Work out the finished part from the listing and answer in its coordinate system (mm). A direction names the side the tool comes from. Round coordinates to 2 decimals unless told otherwise and drop trailing zeros. Loops run counter-clockwise (first coordinate to the right, second up) from the corner with the lowest first, then second, coordinate; pieces in that order, holes last. Notation, with made-up numbers: (25, -37) -> (72, -37) arc R20 ccw to (72, -14) -> close; hole circle Ø7 at (-16.75, 11). An arc over 180 degrees is marked (long way). Use one line per item in the form item = value.
```python
from build123d import *

# Parameters (mm, degrees)
ESQUISSE1_W        = 49.7
ESQUISSE1_H        = 55.3
ESQUISSE1_R        = 2
BOSS_EXTRU_1_DEPTH = 1.5
CONG_1_R           = 1
ESQUISSE2_W        = 24
ESQUISSE2_H        = 10.127456192
BOSS_EXTRU_2_DEPTH = 25
ESQUISSE3_W        = 7.5
ESQUISSE3_H        = 10.5
BOSS_EXTRU_3_DEPTH = 10
ESQUISSE4_W        = 15
ESQUISSE4_H        = 8
BOSS_EXTRU_4_DEPTH = 10
ESQUISSE5_W        = 8
ESQUISSE5_H        = 8
BOSS_EXTRU_5_DEPTH = 8


with BuildPart() as part:
    # Esquisse1 → Boss.-Extru.1 (new body)
    with BuildSketch(Plane.XY):
        with Locations((24.85, 27.65)):
            Rectangle(ESQUISSE1_W, ESQUISSE1_H)
        with Locations((3.6, 51.7)):
            Circle(ESQUISSE1_R, mode=Mode.SUBTRACT)
        with Locations((46.1, 51.7)):
            Circle(ESQUISSE1_R, mode=Mode.SUBTRACT)
        with Locations((46.1, 3.6)):
            Circle(ESQUISSE1_R, mode=Mode.SUBTRACT)
        with Locations((3.6, 3.6)):
            Circle(ESQUISSE1_R, mode=Mode.SUBTRACT)
    extrude(amount=BOSS_EXTRU_1_DEPTH)

    # Congé1
    cong_1_edges = [part.edges().sort_by_distance(p)[0] for p in [
        (0, 55.3, 0.75),
        (49.7, 55.3, 0.75),
        (49.7, 0, 0.75),
        (0, 0, 0.75),
    ]]
    fillet(cong_1_edges, radius=CONG_1_R)

    # Esquisse2 → Boss.-Extru.2 (add)
    with BuildSketch(Plane.XY.offset(1.5)):
        with Locations((24.85, 50.236271904)):
            Rectangle(ESQUISSE2_W, ESQUISSE2_H)
    extrude(amount=BOSS_EXTRU_2_DEPTH)

    # Esquisse3 → Boss.-Extru.3 (add)
    with BuildSketch(Plane.XY.offset(1.5)):
        with Locations((3.75, 17.25)):
            Rectangle(ESQUISSE3_W, ESQUISSE3_H)
        with Locations((45.95, 17.25)):
            Rectangle(ESQUISSE3_W, ESQUISSE3_H)
    extrude(amount=BOSS_EXTRU_3_DEPTH)

    # Esquisse4 → Boss.-Extru.4 (add)
    with BuildSketch(Plane.XY.offset(1.5)):
        with Locations((24.85, 5)):
            Rectangle(ESQUISSE4_W, ESQUISSE4_H)
    extrude(amount=BOSS_EXTRU_4_DEPTH)

    # Esquisse5 → Boss.-Extru.5 (add)
    with BuildSketch(Plane.XY.offset(1.5)):
        with Locations((36.35, 5)):
            Rectangle(ESQUISSE5_W, ESQUISSE5_H)
    extrude(amount=BOSS_EXTRU_5_DEPTH)


solid = part.part
```
(1) Find section B-B, the plane y = 51.7. Write down the section's boundary in (x, z), then the cut area to 3 significant figures.
Completed:
outline = (0, 0) -> (1.6, 0) -> (1.6, 1.5) -> (0, 1.5) -> close; (5.6, 0) -> (44.1, 0) -> (44.1, 1.5) -> (36.85, 1.5) -> (36.85, 26.5) -> (12.85, 26.5) -> (12.85, 1.5) -> (5.6, 1.5) -> close; (48.1, 0) -> (49.7, 0) -> (49.7, 1.5) -> (48.1, 1.5) -> close
area = 663 mm2
(2) For faces 5 (the flat face through (4, 22.5, 6)), 6 (the flat face through (29, 9, 6)), 7 (the flat face through (12.85, 50, 14)), determine the directions among +Z, -Z, +X, -X, +Y, -Y from which every point of the face is accessible in a straight line to the end or side of a thin tool.
Completed:
face_5 = +Z, +X, -X, +Y
face_6 = +Z, +X, -X
face_7 = +Z, -X, +Y, -Y
(3) Find section D-D, the plane x = 28. Write down the section's boundary in (y, z), then the cut area to 3 significant figures.
Completed:
outline = (0, 0) -> (55.3, 0) -> (55.3, 26.5) -> (45.17, 26.5) -> (45.17, 1.5) -> (9, 1.5) -> (9, 11.5) -> (1, 11.5) -> (1, 1.5) -> (0, 1.5) -> close
area = 416 mm2
(4) Consider L1, parallel to Y at x = 46.1, z = 0.9; L2, parallel to X at y = 18, z = 9.5; L3, parallel to Y at x = 32, z = 19.25. Determine where each line is inside the solid, lowest interval first.
Completed:
L1 = 0 to 1.6, 5.6 to 49.7, 53.7 to 55.3
L2 = 0 to 7.5, 42.2 to 49.7
L3 = 45.17 to 55.3
(5) Find section C-C, the plane z = 10.5. Write down the section's boundary in (x, y).
Completed:
outline = (0, 12) -> (7.5, 12) -> (7.5, 22.5) -> (0, 22.5) -> close; (12.85, 45.17) -> (36.85, 45.17) -> (36.85, 55.3) -> (12.85, 55.3) -> close; (17.35, 1) -> (32.35, 1) -> (32.35, 9) -> (17.35, 9) -> close; (42.2, 12) -> (49.7, 12) -> (49.7, 22.5) -> (42.2, 22.5) -> close
(6) For a pull along Y with two mould halves and no side action, classify faces 1 (the flat face through (46, 12, 6)), 2 (the flat face through (46, 22.5, 6)), 3 (the flat face through (25, 28, 1.5)), 4 (the flat face through (42.2, 17, 6)) as +Y half, -Y half, draft (parallel to the pull), parting line (faces both ways), or undercut.
Completed:
face_1 = -Y half
face_2 = +Y half
face_3 = undercut
face_4 = draft
(7) Find section A-A, the plane x = 46.1. Write down the section's boundary in (y, z), then the cut area to 3 significant figures.
Completed:
outline = (0, 0) -> (1.6, 0) -> (1.6, 1.5) -> (0, 1.5) -> close; (5.6, 0) -> (49.7, 0) -> (49.7, 1.5) -> (22.5, 1.5) -> (22.5, 11.5) -> (12, 11.5) -> (12, 1.5) -> (5.6, 1.5) -> close; (53.7, 0) -> (55.3, 0) -> (55.3, 1.5) -> (53.7, 1.5) -> close
area = 176 mm2
(8) Given P1, Ø10, axis at x = 11.5, y = 31.5, coming from the +Z side; P2, Ø2, axis at x = 5.5, z = 8, coming from the -Y side; P3, Ø4, axis at x = 44.5, y = 17, coming from the +Z side; P4, Ø4, axis at x = 34.5, y = 17, coming from the -Z side, each flat-ended and moving along its own axis, determine where each tip first touches the part or whether it passes through.
Completed:
P1 = 1.5
P2 = 12
P3 = 11.5
P4 = 0
